Model file for the job. Use its own axes, mm. A direction names the side the tool comes from. Round coordinates to 2 decimals unless told otherwise and drop trailing zeros. Order: outer loops, then holes, each group sorted by start corner. A loop starts at its lowest first (then second) coordinate and runs counter-clockwise, first axis right, second up. Notation, with made-up numbers: (89, 9) -> (113, 9) arc R27 ccw to (113, 27) -> close; hole circle Ø3 at (-21, -0.75). An arc over 180 degrees is marked (long way). Use CSV: the item, a comma, the result in double quotes.
```python
from build123d import *

# Parameters (mm, degrees)
SZKIC1_R                    = 3
SZKIC1_R_2                  = 0.635
DODANIE_WYCI_GNI_CIE1_DEPTH = 5
SZKIC1_2_R                  = 3
DODANIE_WYCI_GNI_CIE2_DEPTH = 15


with BuildPart() as part:
    # Szkic1 → Dodanie-wyci_gni_cie1 (new body)
    with BuildSketch(Plane.XY):
        with BuildLine():
            Line((-50.67287635, 5.055665151), (-9.235111676, 10.570763761))
            ThreePointArc((-9.235111676, 10.570763761), (0, 11.182632843), (9.235111676, 10.570763761))
            Line((9.235111676, 10.570763761), (50.67287635, 5.055665151))
            ThreePointArc((50.67287635, 5.055665151), (55.100246338, 0), (50.67287635, -5.055665151))
            Line((50.67287635, -5.055665151), (9.235111676, -10.570763761))
            ThreePointArc((9.235111676, -10.570763761), (0, -11.182632843), (-9.235111676, -10.570763761))
            Line((-9.235111676, -10.570763761), (-50.67287635, -5.055665151))
            ThreePointArc((-50.67287635, -5.055665151), (-55.100246338, 0), (-50.67287635, 5.055665151))
        make_face()
        Circle(SZKIC1_R, mode=Mode.SUBTRACT)
        with Locations((-5.656854249, 5.656854249)):
            Circle(SZKIC1_R_2, mode=Mode.SUBTRACT)
        with Locations((-8, 0)):
            Circle(SZKIC1_R_2, mode=Mode.SUBTRACT)
        with Locations((0, 8)):
            Circle(SZKIC1_R_2, mode=Mode.SUBTRACT)
        with Locations((5.656854249, 5.656854249)):
            Circle(SZKIC1_R_2, mode=Mode.SUBTRACT)
        with Locations((-50, 0)):
            Circle(SZKIC1_R, mode=Mode.SUBTRACT)
        with Locations((50, 0)):
            Circle(SZKIC1_R, mode=Mode.SUBTRACT)
        with Locations((8, 0)):
            Circle(SZKIC1_R_2, mode=Mode.SUBTRACT)
        with Locations((5.656854249, -5.656854249)):
            Circle(SZKIC1_R_2, mode=Mode.SUBTRACT)
        with Locations((0, -8)):
            Circle(SZKIC1_R_2, mode=Mode.SUBTRACT)
        with Locations((-5.656854249, -5.656854249)):
            Circle(SZKIC1_R_2, mode=Mode.SUBTRACT)
    extrude(amount=DODANIE_WYCI_GNI_CIE1_DEPTH)

    # Szkic1_2 → Dodanie-wyci_gni_cie2 (add)
    with BuildSketch(Plane.XY):
        with Locations((-50, 0)):
            Circle(SZKIC1_2_R)
        with Locations((50, 0)):
            Circle(SZKIC1_2_R)
    extrude(amount=DODANIE_WYCI_GNI_CIE2_DEPTH)


solid = part.part
```
Q1. Cut at B-B (y = 1.75). Give the cut face in (x, z).
From the geometry:
outline,"(-54.79, 0) -> (-2.44, 0) -> (-2.44, 5) -> (-47.56, 5) -> (-47.56, 15) -> (-52.44, 15) -> (-52.44, 5) -> (-54.79, 5) -> close; (2.44, 0) -> (54.79, 0) -> (54.79, 5) -> (52.44, 5) -> (52.44, 15) -> (47.56, 15) -> (47.56, 5) -> (2.44, 5) -> close"
Q2. Which spindle directions (+Z, -Z, +X, -X, +Y, -Y) get a long thin tool onto all of the face, cutting with end or side? Do faces 1 (the cylindrical face through (47, 0, 10)), 2 (the flat face through (-50, 0, 15)). Say none if no direction does.
From the geometry:
face 1,"+Z"
face 2,"+Z, +X, -X, +Y, -Y"
Q3. Probe line 1 along Z through (x, y) = (33, -6.75); line 2 along X through (y, z) = (0.5, 13.5); line 3 along Y through (x, z) = (10, 3.5). List the from-to ranges inside material, lowest first.
From the geometry:
line 1,"z = 0 to 5"
line 2,"x = -52.96 to -47.04, 47.04 to 52.96"
line 3,"y = -10.47 to 10.47"
Q4. Pin check, flat tips, straight feed: pin 1 (12 mm diameter, centred on x = -31.5, y = -2.5, fed in from +Z); pin 2 (1.5 mm diameter, centred on x = 28.5, z = 5.5, fed in from +Y). Stop position of each tip, or through.
From the geometry:
pin 1,"stops at z = 5"
pin 2,"stops at y = 8.08"
Q5. Cut at C-C (x = 37). Give the cut face in (y, z), plus the area to 3 significant figures.
From the geometry:
outline,"(-6.88, 0) -> (6.88, 0) -> (6.88, 5) -> (-6.88, 5) -> close"
area,"68.8 mm²"
Q6. Cut at A-A (z = 13.25). Give the cut face in (x, y).
From the geometry:
outline,"circle Ø6 at (-50, 0); circle Ø6 at (50, 0)"
Q7. Mould opens along X. For faces 3 (the flat face through (30.244, -7.775, 2.465)), 4 (the cylindrical face through (0.13, -11.183, 2.465)), 5 (the cylindrical face through (-53, 0, 10)) say: +X half, -X half, draft (parallel to the pull), parting line (faces both ways), or undercut.
From the geometry:
face 3,"+X half"
face 4,"parting line"
face 5,"undercut"
Q8. Cut at D-D (x = -29). Give the cut face in (y, z).
From the geometry:
outline,"(-7.94, 0) -> (7.94, 0) -> (7.94, 5) -> (-7.94, 5) -> close"
